```python
from build123d import *

# Parameters (mm, degrees)
FILLET1_R = 1


with BuildPart() as part:
    # Sketch1 → Revolve1 (revolve)
    with BuildSketch(Plane(origin=(0, 0, 0), x_dir=(1, 0, 0), z_dir=(0, 1, 0)), mode=Mode.PRIVATE) as revolve1_sk:
        with BuildLine():
            Line((0, 0), (61.160254038, 0))
            Line((61.160254038, 0), (61.160254038, 8))
            Line((61.160254038, 8), (11.160254038, 8))
            Line((11.160254038, 8), (11.160254038, 3.5))
            ThreePointArc((11.160254038, 3.5), (10.940584124, 2.969669914), (10.410254038, 2.75))
            Line((10.410254038, 2.75), (9.410254038, 2.75))
            ThreePointArc((9.410254038, 2.75), (8.879923952, 2.969669914), (8.660254038, 3.5))
            Line((8.660254038, 3.5), (8.660254038, 5))
            ThreePointArc((8.660254038, 5), (-2.588190451, 9.659258263), (-10, 0))
            Line((-10, 0), (0, 0))
        make_face()
    revolve(revolve1_sk.sketch.rotate(Axis((0, 0, 0), (1, 0, 0)), 180), axis=Axis((0, 0, 0), (1, 0, 0)))

    # Fillet1
    fillet1_edges = [part.edges().sort_by_distance(p)[0] for p in [
        (61.160254038, 0, -8),
        (11.160254038, 0, -8),
    ]]
    fillet(fillet1_edges, radius=FILLET1_R)


solid = part.part
```
The model under review builds one solid part; all positions refer to its coordinate system, in mm. Give positions to 0.01 mm unless a question says otherwise; leave off trailing zeros. Write each loop counter-clockwise with the first axis right and the second up, starting at its lowest first coordinate (ties: lowest second). Pieces come first, ordered by that corner, then holes. Notation, with made-up numbers: M -23.75,13 L 21.25,13 A29 ccw 21.25,47 Z; hole C 37,88.25 d9. An arc over 180 degrees is marked long. Write item = value, one per line. Start each with the question number.
Q1. Clearance check with flat-ended pins moving along their axes: pin 1 (1.5 mm diameter, centred on x = 2.5, y = -0.5, fed in from -Z); pin 2 (8 mm diameter, centred on y = 1.5, z = 7.5, fed in from +X); pin 3 (10 mm diameter, centred on x = 2, y = -6, fed in from -Z); pin 4 (6 mm diameter, centred on y = 7, z = -3, fed in from -X). State where each tip first meets the part, or that it passes through.
Q2. We need section A-A (z = 0). State the section outline as (x, y) points, plus the area to 3 significant figures.
Q3. We need section D-D (x = 5). State the section outline as (y, z) points.
Q4. We need section C-C (x = 55). State the section outline as (y, z) points, plus the area to 3 significant figures.
Q5. For line 1 (X direction, y = -4.75, z = -2.75); line 2 (X direction, y = 5, z = 0); line 3 (X direction, y = 4, z = 8.25), list the stretches that pass through material, from the lowest coordinate up.
Q6. Mouldability with a two-part tool opening along X and no side actions: class faces 1 (the face through (9.903, 2.685, -0.596)), 2 (the face through (35.82, 7.81, -1.73)), 3 (the face through (61.16, 0, 0)) as released by +X, released by -X, zero draft, split by the parting line, or undercut.
Result set:
q1.pin_1 = -9.84
q1.pin_2 = 61.16
q1.pin_3 = -9.91
q1.pin_4 = -8.87
q2.outline = M 8.66,-5 L 8.66,-3.5 A0.75 cw 9.41,-2.75 L 10.41,-2.75 A0.75 cw 11.16,-3.5 L 11.16,-7 A1 ccw 12.16,-8 L 60.16,-8 A1 ccw 61.16,-7 L 61.16,7 A1 ccw 60.16,8 L 12.16,8 A1 ccw 11.16,7 L 11.16,3.5 A0.75 cw 10.41,2.75 L 9.41,2.75 A0.75 cw 8.66,3.5 L 8.66,5 A10 ccw long Z
q2.area = 1,120 mm2
q3.outline = C 0,0 d17.32
q4.outline = C 0,0 d16
q4.area = 201 mm2
q5.line_1 = -8.36 to 8.36, 11.16 to 61.16
q5.line_2 = -8.66 to 8.66, 11.16 to 61.16
q5.line_3 = -3.99 to 3.99
q6.face_1 = undercut
q6.face_2 = zero draft
q6.face_3 = released by +X
